Source: CAD feature listing. Evaluate the final solid. Frame: model axes, mm. Round coordinates to 2 decimals unless told otherwise and drop trailing zeros. Order: outer loops, then holes, each group sorted by start corner. A loop starts at its lowest first (then second) coordinate and runs counter-clockwise, first axis right, second up. Notation, with made-up numbers: (49.5, 33) - (108.5, 33) arc R6 cw to (108.5, 44) - close; hole circle Ø4 at (22, 47). An arc over 180 degrees is marked (long way). Return JSON: item names as keys, results as strings. Group by question number.
1) Contact query for a flat-ended pin moving along its axis: P1, Ø3, axis at x = -610.1, y = -42.14, coming from the +Z side. Output: stop coordinate, or through.
2) Ray query, line 1 (X direction, y = -122.5, z = 0.85); line 2 (X direction, y = 9.5, z = 0.8); line 3 (Y direction, x = 527, z = 1.45). Return the intervals inside material, ascending. Write a range as from..to.
3) Section A-A, the plane x = 525.5. Return loops of the section in (y, z), plus the area to 3 significant figures.
4) Section B-B, the plane z = 0.85. Give the number of separate pieces and of enclosed holes in the cut face, plus the area to 3 significant figures.
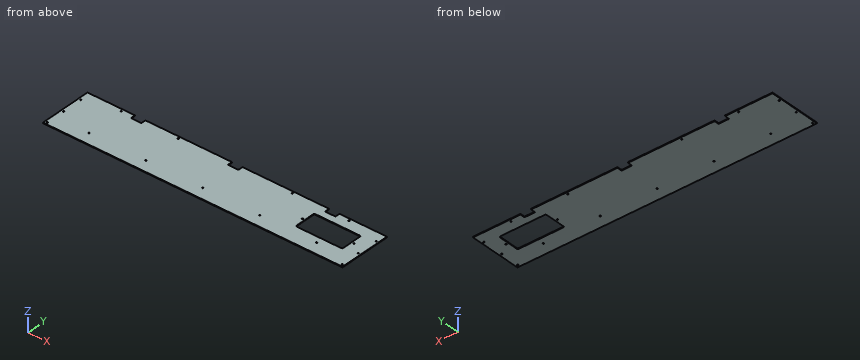
```python
from build123d import *

# Parameters (mm, degrees)
SKETCH1_R           = 2.55
BOSS_EXTRUDE1_DEPTH = 3


with BuildPart() as part:
    # Sketch1 → Boss-Extrude1 (new body)
    with BuildSketch(Plane.XY):
        Polygon((431.898025048, 87.861768757), (629.898025048, 87.861768757), (629.898025048, -132.138231243), (-620.101974952, -132.138231243), (-620.101974952, 87.861768757), (-422.101974952, 87.861768757), (-422.101974952, 67.861768757), (-378.101974952, 67.861768757), (-378.101974952, 87.861768757), (-17.101974952, 87.861768757), (-17.101974952, 67.861768757), (26.898025048, 67.861768757), (26.898025048, 87.861768757), (387.898025048, 87.861768757), (387.898025048, 67.861768757), (431.898025048, 67.861768757), align=None)
        with Locations((242.398025048, 77.861768757)):
            Circle(SKETCH1_R, mode=Mode.SUBTRACT)
        with Locations((-610.101974952, 42.861768757)):
            Circle(SKETCH1_R, mode=Mode.SUBTRACT)
        with Locations((-232.601974952, 77.861768757)):
            Circle(SKETCH1_R, mode=Mode.SUBTRACT)
        with Locations((-470.101974952, 77.861768757)):
            Circle(SKETCH1_R, mode=Mode.SUBTRACT)
        with Locations((479.898025048, 77.861768757)):
            Circle(SKETCH1_R, mode=Mode.SUBTRACT)
        with Locations((479.898025048, -82.138231243)):
            Circle(SKETCH1_R, mode=Mode.SUBTRACT)
        with Locations((242.398025048, -82.138231243)):
            Circle(SKETCH1_R, mode=Mode.SUBTRACT)
        with Locations((4.898025048, -82.138231243)):
            Circle(SKETCH1_R, mode=Mode.SUBTRACT)
        with Locations((-232.601974952, -82.138231243)):
            Circle(SKETCH1_R, mode=Mode.SUBTRACT)
        with Locations((-470.101974952, -82.138231243)):
            Circle(SKETCH1_R, mode=Mode.SUBTRACT)
        with Locations((619.898025048, -42.138231243)):
            Circle(SKETCH1_R, mode=Mode.SUBTRACT)
        with Locations((-610.101974952, -42.138231243)):
            Circle(SKETCH1_R, mode=Mode.SUBTRACT)
        with Locations((-610, -122.138231243)):
            Circle(SKETCH1_R, mode=Mode.SUBTRACT)
        with Locations((619.898025048, 45.705315607)):
            Circle(SKETCH1_R, mode=Mode.SUBTRACT)
        with Locations((619.898025048, -122.138231243)):
            Circle(SKETCH1_R, mode=Mode.SUBTRACT)
        with Locations((574.10958906, -9.140897424)):
            Circle(SKETCH1_R, mode=Mode.SUBTRACT)
        with Locations((359.10958906, -9.140897424)):
            Circle(SKETCH1_R, mode=Mode.SUBTRACT)
        with BuildLine():
            Line((559.10958906, 36.859102576), (374.10958906, 36.859102576))
            ThreePointArc((374.10958906, 36.859102576), (370.574055154, 35.394636482), (369.10958906, 31.859102576))
            Line((369.10958906, 31.859102576), (369.10958906, -50.140897424))
            ThreePointArc((369.10958906, -50.140897424), (370.574055154, -53.67643133), (374.10958906, -55.140897424))
            Line((374.10958906, -55.140897424), (559.10958906, -55.140897424))
            ThreePointArc((559.10958906, -55.140897424), (562.645122966, -53.67643133), (564.10958906, -50.140897424))
            Line((564.10958906, -50.140897424), (564.10958906, 31.859102576))
            ThreePointArc((564.10958906, 31.859102576), (562.645122966, 35.394636482), (559.10958906, 36.859102576))
        make_face(mode=Mode.SUBTRACT)
    extrude(amount=BOSS_EXTRUDE1_DEPTH)


solid = part.part
```
Geometry check:
{
 "1": {"P1": "through"},
 "2": {"line 1": "-620.1..-612.52, -607.48..617.37, 622.42..629.9", "line 2": "-620.1..369.11, 564.11..629.9", "line 3": "-132.14..-55.14, 36.86..87.86"},
 "3": {"outline": "(-132.14, 0) - (-55.14, 0) - (-55.14, 3) - (-132.14, 3) - close; (36.86, 0) - (87.86, 0) - (87.86, 3) - (36.86, 3) - close", "area": "384 mm2"},
 "4": {"separate pieces": "1", "enclosed holes": "18", "area": "254,000 mm2"}
}
